Could you check a few things on this drawing? It's one solid part, dimensions in mm from its lowest x, y, z. A direction names the side the tool comes from. Round coordinates to 2 decimals unless told otherwise and drop trailing zeros. Order: outer loops, then holes, each group sorted by start corner. A loop starts at its lowest first (then second) coordinate and runs counter-clockwise, first axis right, second up. Notation, with made-up numbers: (-21.5, 66.5) - (12.5, 66.5) arc R15 cw to (12.5, 80.5) - close; hole circle Ø11 at (6, 20). An arc over 180 degrees is marked (long way). Use one line per item in the form item = value.
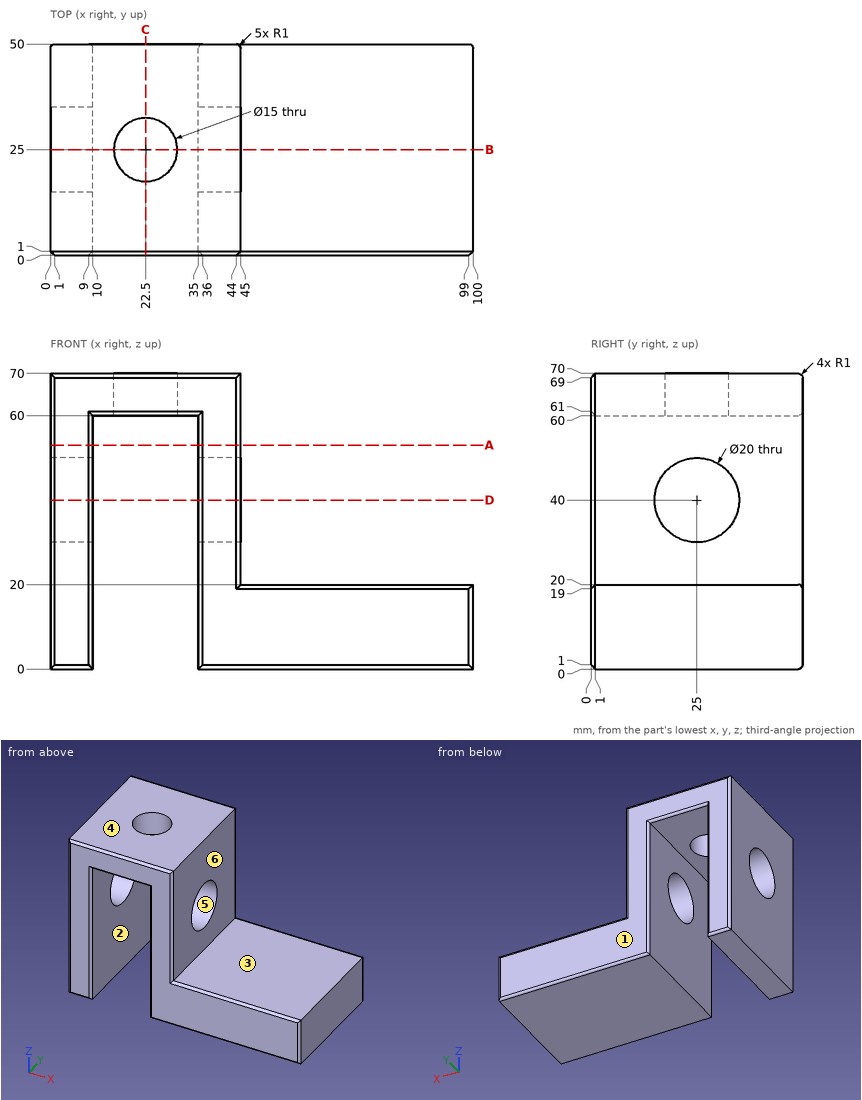
Item 1: For the marked faces 1, 2 and 3, which set-ups out of +Z, -Z, +X, -X, +Y, -Y let a thin tool reach every point of the face, with its end or its side?
Found:
face_1 = +Z, -Z, +X, -X, +Y
face_2 = -Z, +Y, -Y
face_3 = +Z, +X, +Y, -Y
Item 2: If we mould it in two halves opening along Z, with no side actions, what happens to the marked faces 4, 5 and 6? For each: released by +Z, released by -Z, zero draft, split by the parting line, or undercut.
Found:
face_4 = released by +Z
face_5 = undercut
face_6 = zero draft
Item 3: Imagine slicing it at B-B on y = 25. Please give me the cut outline in (x, z), plus the area to 3 significant figures.
Found:
outline = (0, 0) - (10, 0) - (10, 30) - (0, 30) - close; (0, 50) - (10, 50) - (10, 60) - (15, 60) - (15, 70) - (0, 70) - close; (30, 60) - (35, 60) - (35, 50) - (45, 50) - (45, 70) - (30, 70) - close; (35, 0) - (100, 0) - (100, 20) - (45, 20) - (45, 30) - (35, 30) - close
area = 2,200 mm2
Item 4: Imagine slicing it at C-C on x = 22.5. Please give me the cut outline in (y, z), plus the area to 3 significant figures.
Found:
outline = (0, 61) - (1, 60) - (17.5, 60) - (17.5, 70) - (1, 70) - (0, 69) - close; (32.5, 60) - (49, 60) arc R1 ccw to (50, 61) - (50, 69) arc R1 ccw to (49, 70) - (32.5, 70) - close
area = 349 mm2
Item 5: Imagine slicing it at A-A on z = 53. Please give me the cut outline in (x, y).
Found:
outline = (0, 1) - (1, 0) - (9, 0) - (10, 1) - (10, 49) arc R1 ccw to (9, 50) - (1, 50) arc R1 ccw to (0, 49) - close; (35, 1) - (36, 0) - (44, 0) - (45, 1) - (45, 49) arc R1 ccw to (44, 50) - (36, 50) arc R1 ccw to (35, 49) - close
Item 6: Imagine slicing it at D-D on z = 40. Please give me the cut outline in (x, y), plus the area to 3 significant figures.
Found:
outline = (0, 1) - (1, 0) - (9, 0) - (10, 1) - (10, 15) - (0, 15) - close; (0, 35) - (10, 35) - (10, 49) arc R1 ccw to (9, 50) - (1, 50) arc R1 ccw to (0, 49) - close; (35, 1) - (36, 0) - (44, 0) - (45, 1) - (45, 15) - (35, 15) - close; (35, 35) - (45, 35) - (45, 49) arc R1 ccw to (44, 50) - (36, 50) arc R1 ccw to (35, 49) - close
area = 597 mm2
Item 7: I need wall thicknesses on L1, parallel to Z at x = 43, y = 25; L2, parallel to X at y = 40.5, z = 33.5; L3, parallel to X at y = 17, z = 17. Which ranges of each line are inside material? Lowest first, please.
Found:
L1 = 0 to 30, 50 to 70
L2 = 0 to 10, 35 to 45
L3 = 0 to 10, 35 to 100
Item 8: Will these pins go through, and if not, where does the flat tip stop? P1, Ø4, axis at y = 14.5, z = 26, coming from the +X side; P2, Ø16, axis at y = 25, z = 40, coming from the -X side; P3, Ø8, axis at x = 19.5, y = 12.5, coming from the -Z side.
Found:
P1 = 45
P2 = through
P3 = 60
